```python
from build123d import *

# Parameters (mm, degrees)
SKETCH3_W           = 22
SKETCH3_H           = 5.7785
BOSS_EXTRUDE2_DEPTH = 101
CUT_EXTRUDE1_DEPTH  = 104.529662717
FILLET1_R           = 1.2637
SKETCH10_W          = 101
SKETCH10_H          = 62
BOSS_EXTRUDE6_DEPTH = 8
SKETCH11_R          = 2.5
CUT_EXTRUDE2_DEPTH  = 110.676797911
SKETCH12_R          = 2.5
CUT_EXTRUDE3_DEPTH  = 110.676797911


with BuildPart() as part:
    # Sketch3 → Boss-Extrude2 (new body)
    with BuildSketch(Plane(origin=(0, 0, 0), x_dir=(0, 0, -1), z_dir=(1, 0, 0))):
        with Locations((11, 2.88925)):
            Rectangle(SKETCH3_W, SKETCH3_H)
    extrude(amount=-BOSS_EXTRUDE2_DEPTH)

    # Sketch5 → Cut-Extrude1 (cut, through all)
    with BuildSketch(Plane(origin=(0, 0, 0), x_dir=(-1, 0, 0), z_dir=(0, 0, -1))):
        with BuildLine():
            Line((1.674138493, 2.258445519), (0.421264214, 6.934235985))
            Line((0.421264214, 6.934235985), (6.147128546, 6.934235985))
            Line((6.147128546, 6.934235985), (4.894261507, 2.258445519))
            ThreePointArc((4.894261507, 2.258445519), (4.454663567, 1.600540709), (3.7054, 1.3462))
            Line((3.7054, 1.3462), (2.863, 1.3462))
            ThreePointArc((2.863, 1.3462), (2.113736433, 1.600540709), (1.674138493, 2.258445519))
        make_face()
        with BuildLine():
            Line((10.263138493, 2.258445519), (9.010264214, 6.934235985))
            Line((9.010264214, 6.934235985), (14.736128546, 6.934235985))
            Line((14.736128546, 6.934235985), (13.483261507, 2.258445519))
            ThreePointArc((13.483261507, 2.258445519), (13.043663567, 1.600540709), (12.2944, 1.3462))
            Line((12.2944, 1.3462), (11.452, 1.3462))
            ThreePointArc((11.452, 1.3462), (10.702736433, 1.600540709), (10.263138493, 2.258445519))
        make_face()
        with BuildLine():
            Line((18.852138493, 2.258445519), (17.599264214, 6.934235985))
            Line((17.599264214, 6.934235985), (23.325128546, 6.934235985))
            Line((23.325128546, 6.934235985), (22.072261507, 2.258445519))
            ThreePointArc((22.072261507, 2.258445519), (21.632663567, 1.600540709), (20.8834, 1.3462))
            Line((20.8834, 1.3462), (20.041, 1.3462))
            ThreePointArc((20.041, 1.3462), (19.291736433, 1.600540709), (18.852138493, 2.258445519))
        make_face()
        with BuildLine():
            Line((27.441138493, 2.258445519), (26.188264214, 6.934235985))
            Line((26.188264214, 6.934235985), (31.914128546, 6.934235985))
            Line((31.914128546, 6.934235985), (30.661261507, 2.258445519))
            ThreePointArc((30.661261507, 2.258445519), (30.221663567, 1.600540709), (29.4724, 1.3462))
            Line((29.4724, 1.3462), (28.63, 1.3462))
            ThreePointArc((28.63, 1.3462), (27.880736433, 1.600540709), (27.441138493, 2.258445519))
        make_face()
        with BuildLine():
            Line((36.030138493, 2.258445519), (34.777264214, 6.934235985))
            Line((34.777264214, 6.934235985), (40.503128546, 6.934235985))
            Line((40.503128546, 6.934235985), (39.250261507, 2.258445519))
            ThreePointArc((39.250261507, 2.258445519), (38.810663567, 1.600540709), (38.0614, 1.3462))
            Line((38.0614, 1.3462), (37.219, 1.3462))
            ThreePointArc((37.219, 1.3462), (36.469736433, 1.600540709), (36.030138493, 2.258445519))
        make_face()
        with BuildLine():
            Line((44.619138493, 2.258445519), (43.366264214, 6.934235985))
            Line((43.366264214, 6.934235985), (49.092128546, 6.934235985))
            Line((49.092128546, 6.934235985), (47.839261507, 2.258445519))
            ThreePointArc((47.839261507, 2.258445519), (47.399663567, 1.600540709), (46.6504, 1.3462))
            Line((46.6504, 1.3462), (45.808, 1.3462))
            ThreePointArc((45.808, 1.3462), (45.058736433, 1.600540709), (44.619138493, 2.258445519))
        make_face()
        with BuildLine():
            Line((53.208138493, 2.258445519), (51.955264214, 6.934235985))
            Line((51.955264214, 6.934235985), (57.681128546, 6.934235985))
            Line((57.681128546, 6.934235985), (56.428261507, 2.258445519))
            ThreePointArc((56.428261507, 2.258445519), (55.988663567, 1.600540709), (55.2394, 1.3462))
            Line((55.2394, 1.3462), (54.397, 1.3462))
            ThreePointArc((54.397, 1.3462), (53.647736433, 1.600540709), (53.208138493, 2.258445519))
        make_face()
        with BuildLine():
            Line((61.797138493, 2.258445519), (60.544264214, 6.934235985))
            Line((60.544264214, 6.934235985), (66.270128546, 6.934235985))
            Line((66.270128546, 6.934235985), (65.017261507, 2.258445519))
            ThreePointArc((65.017261507, 2.258445519), (64.577663567, 1.600540709), (63.8284, 1.3462))
            Line((63.8284, 1.3462), (62.986, 1.3462))
            ThreePointArc((62.986, 1.3462), (62.236736433, 1.600540709), (61.797138493, 2.258445519))
        make_face()
        with BuildLine():
            Line((70.386138493, 2.258445519), (69.133264214, 6.934235985))
            Line((69.133264214, 6.934235985), (74.859128546, 6.934235985))
            Line((74.859128546, 6.934235985), (73.606261507, 2.258445519))
            ThreePointArc((73.606261507, 2.258445519), (73.166663567, 1.600540709), (72.4174, 1.3462))
            Line((72.4174, 1.3462), (71.575, 1.3462))
            ThreePointArc((71.575, 1.3462), (70.825736433, 1.600540709), (70.386138493, 2.258445519))
        make_face()
        with BuildLine():
            Line((78.975138493, 2.258445519), (77.722264214, 6.934235985))
            Line((77.722264214, 6.934235985), (83.448128546, 6.934235985))
            Line((83.448128546, 6.934235985), (82.195261507, 2.258445519))
            ThreePointArc((82.195261507, 2.258445519), (81.755663567, 1.600540709), (81.0064, 1.3462))
            Line((81.0064, 1.3462), (80.164, 1.3462))
            ThreePointArc((80.164, 1.3462), (79.414736433, 1.600540709), (78.975138493, 2.258445519))
        make_face()
        with BuildLine():
            Line((87.564138493, 2.258445519), (86.311264214, 6.934235985))
            Line((86.311264214, 6.934235985), (92.037128546, 6.934235985))
            Line((92.037128546, 6.934235985), (90.784261507, 2.258445519))
            ThreePointArc((90.784261507, 2.258445519), (90.344663567, 1.600540709), (89.5954, 1.3462))
            Line((89.5954, 1.3462), (88.753, 1.3462))
            ThreePointArc((88.753, 1.3462), (88.003736433, 1.600540709), (87.564138493, 2.258445519))
        make_face()
        with BuildLine():
            Line((96.153138493, 2.258445519), (94.900264214, 6.934235985))
            Line((94.900264214, 6.934235985), (100.626128546, 6.934235985))
            Line((100.626128546, 6.934235985), (99.373261507, 2.258445519))
            ThreePointArc((99.373261507, 2.258445519), (98.933663567, 1.600540709), (98.1844, 1.3462))
            Line((98.1844, 1.3462), (97.342, 1.3462))
            ThreePointArc((97.342, 1.3462), (96.592736433, 1.600540709), (96.153138493, 2.258445519))
        make_face()
    extrude(amount=CUT_EXTRUDE1_DEPTH, mode=Mode.SUBTRACT)

    # Fillet1
    # the kernel refuses this fillet: 1.2637 mm, written as the material it takes off along each edge
    with BuildSketch(Plane(origin=(-14.426451812, 5.7785, -24.424181413), x_dir=(-1, 0, 0), z_dir=(0, 0, 1)), Plane(origin=(-23.015451812, 5.7785, -24.424181413), x_dir=(-1, 0, 0), z_dir=(0, 0, 1)), Plane(origin=(-31.604451812, 5.7785, -24.424181413), x_dir=(-1, 0, 0), z_dir=(0, 0, 1)), Plane(origin=(-40.193451812, 5.7785, -24.424181413), x_dir=(-1, 0, 0), z_dir=(0, 0, 1)), Plane(origin=(-48.782451812, 5.7785, -24.424181413), x_dir=(-1, 0, 0), z_dir=(0, 0, 1)), Plane(origin=(-57.371451812, 5.7785, -24.424181413), x_dir=(-1, 0, 0), z_dir=(0, 0, 1)), Plane(origin=(-65.960451812, 5.7785, -24.424181413), x_dir=(-1, 0, 0), z_dir=(0, 0, 1)), Plane(origin=(-74.549451812, 5.7785, -24.424181413), x_dir=(-1, 0, 0), z_dir=(0, 0, 1)), Plane(origin=(-83.138451812, 5.7785, -24.424181413), x_dir=(-1, 0, 0), z_dir=(0, 0, 1)), Plane(origin=(-91.727451812, 5.7785, -24.424181413), x_dir=(-1, 0, 0), z_dir=(0, 0, 1)), Plane(origin=(-5.837451812, 5.7785, -24.424181413), x_dir=(-1, 0, 0), z_dir=(0, 0, 1))) as fillet1_piece_1:
        with BuildLine():
            CenterArc((FILLET1_R * 0.767328135667, FILLET1_R), FILLET1_R, 194.999917223, 75.000082777)
            Line((-FILLET1_R * 0.198598064545, FILLET1_R * 0.7411823504), (-FILLET1_R * 0.217916588549, FILLET1_R * 0.736005997408))
            Line((-FILLET1_R * 0.217916588549, FILLET1_R * 0.736005997408), (-FILLET1_R * 0.0153465627133, -FILLET1_R * 0.02))
            Line((-FILLET1_R * 0.0153465627133, -FILLET1_R * 0.02), (FILLET1_R * 0.767328135667, -FILLET1_R * 0.02))
            Line((FILLET1_R * 0.767328135667, -FILLET1_R * 0.02), (FILLET1_R * 0.767328135667, 0))
        make_face()
    extrude(amount=26.848362825, mode=Mode.SUBTRACT)
    with BuildSketch(Plane(origin=(-9.319942738, 5.7785, 2.424177787), x_dir=(-0.25881904510252474, -0.9659258262890672, 0), z_dir=(0, 0, -1)), Plane(origin=(-17.908942738, 5.7785, 2.424177787), x_dir=(-0.25881904510252474, -0.9659258262890672, 0), z_dir=(0, 0, -1)), Plane(origin=(-26.497942738, 5.7785, 2.424177787), x_dir=(-0.25881904510252496, -0.9659258262890672, 0), z_dir=(0, 0, -1)), Plane(origin=(-35.086942738, 5.7785, 2.424177787), x_dir=(-0.2588190451025256, -0.965925826289067, 0), z_dir=(0, 0, -1)), Plane(origin=(-43.675942738, 5.7785, 2.424177787), x_dir=(-0.2588190451025256, -0.965925826289067, 0), z_dir=(0, 0, -1)), Plane(origin=(-52.264942738, 5.7785, 2.424177787), x_dir=(-0.25881904510252424, -0.9659258262890673, 0), z_dir=(0, 0, -1)), Plane(origin=(-60.853942738, 5.7785, 2.424177787), x_dir=(-0.25881904510252424, -0.9659258262890673, 0), z_dir=(0, 0, -1)), Plane(origin=(-69.442942738, 5.7785, 2.424177787), x_dir=(-0.25881904510252607, -0.9659258262890669, 0), z_dir=(0, 0, -1)), Plane(origin=(-78.031942738, 5.7785, 2.424177787), x_dir=(-0.25881904510252607, -0.9659258262890669, 0), z_dir=(0, 0, -1)), Plane(origin=(-86.620942738, 5.7785, 2.424177787), x_dir=(-0.2588190451025252, -0.9659258262890671, 0), z_dir=(0, 0, -1)), Plane(origin=(-95.209942738, 5.7785, 2.424177787), x_dir=(-0.2588190451025268, -0.9659258262890666, 0), z_dir=(0, 0, -1))) as fillet1_piece_2:
        with BuildLine():
            CenterArc((FILLET1_R * 0.767326987979, -FILLET1_R), FILLET1_R, 90, 75)
            Line((-FILLET1_R * 0.19859883831, -FILLET1_R * 0.741180954897), (-FILLET1_R * 0.217917354836, -FILLET1_R * 0.736004573995))
            Line((-FILLET1_R * 0.217917354836, -FILLET1_R * 0.736004573995), (-FILLET1_R * 0.0153465397596, FILLET1_R * 0.02))
            Line((-FILLET1_R * 0.0153465397596, FILLET1_R * 0.02), (FILLET1_R * 0.767326987979, FILLET1_R * 0.02))
            Line((FILLET1_R * 0.767326987979, FILLET1_R * 0.02), (FILLET1_R * 0.767326987979, 0))
        make_face()
    extrude(amount=26.848355574, mode=Mode.SUBTRACT)
    with BuildSketch(Plane(origin=(-100.316451812, 5.7785, -24.33349599), x_dir=(-1, 0, 0), z_dir=(0, 0, 1))) as fillet1_piece_3:
        with BuildLine():
            CenterArc((0.97906096, 1.22866183), FILLET1_R, 194.999917223, 61.476400821)
            Line((-0.241579979, 0.901593966), (-0.265992798, 0.895052609))
            Line((-0.265992798, 0.895052609), (-0.024412819, -0.006541357))
            Line((-0.024412819, -0.006541357), (0, -0.025274))
            ThreePointArc((0, -0.025274), (0.341774094, -0.025274), (0.677637933, -0.024573237))
            Line((0.677637933, -0.024573237), (0.683548188, 0))
        make_face()
    extrude(amount=26.666991979, mode=Mode.SUBTRACT)
    with BuildSketch(Plane(origin=(-0.730942738, 5.7785, 2.362037613), x_dir=(-0.2588190451025249, -0.9659258262890672, 0), z_dir=(0, 0, -1))) as fillet1_piece_4:
        with BuildLine():
            CenterArc((0.944815045, -1.2637), FILLET1_R, 90, 63.813512011)
            Line((-0.189181901, -0.706036468), (-0.21186184, -0.694883197))
            ThreePointArc((-0.21186184, -0.694883197), (-0.11900376, -0.346476841), (-0.024412809, 0.006541393))
            Line((-0.024412809, 0.006541393), (0, 0.025274))
            Line((0, 0.025274), (0.944815045, 0.025274))
            Line((0.944815045, 0.025274), (0.944815045, 0))
        make_face()
    extrude(amount=26.724075226, mode=Mode.SUBTRACT)

    # Sketch10 → Boss-Extrude6 (add)
    with BuildSketch(Plane(origin=(0, 0, 0), x_dir=(1, 0, 0), z_dir=(0, 1, 0))):
        with Locations((-50.5, 11)):
            Rectangle(SKETCH10_W, SKETCH10_H)
    extrude(amount=-BOSS_EXTRUDE6_DEPTH)

    # Sketch11 → Cut-Extrude2 (cut, through all)
    with BuildSketch(Plane(origin=(0, 0, 0), x_dir=(1, 0, 0), z_dir=(0, 1, 0))):
        with Locations(Location((-8.5, -10, 0), (0, 0, 270))):
            Circle(SKETCH11_R)
        with Locations(Location((-92.5, -10, 0), (0, 0, 270))):
            Circle(SKETCH11_R)
    extrude(amount=-CUT_EXTRUDE2_DEPTH, mode=Mode.SUBTRACT)

    # Sketch12 → Cut-Extrude3 (cut, through all)
    with BuildSketch(Plane(origin=(0, 0, 0), x_dir=(1, 0, 0), z_dir=(0, 1, 0))):
        with Locations(Location((-8.5, 32, 0), (0, 0, 270))):
            Circle(SKETCH12_R)
        with Locations(Location((-92.5, 32, 0), (0, 0, 270))):
            Circle(SKETCH12_R)
    extrude(amount=-CUT_EXTRUDE3_DEPTH, mode=Mode.SUBTRACT)


solid = part.part
```
The listing builds one solid part. Answer for the finished solid, in the listing's coordinates (mm). A direction names the side the tool comes from. Coordinates: 2 decimals unless noted, no trailing zeros. Loops run counter-clockwise (first coordinate to the right, second up) from the corner with the lowest first, then second, coordinate; pieces in that order, holes last. Notation, with made-up numbers: (-27, 71) - (-7, 71) arc R11 cw to (-7, 81) - close; hole circle Ø10 at (42.25, -23.75). An arc over 180 degrees is marked (long way). Use a Markdown table: item, result. Add a question column.
1) The part is cut by section B-B, the plane z = 14.5. Give the vertices of the cut face in (x, y).
2) Given pin 1 (0.9 mm diameter, centred on x = -3.5, z = -8, fed in from +Y); pin 2 (4.5 mm diameter, centred on x = -8.5, z = 10, fed in from +Y); pin 3 (22 mm diameter, centred on x = -54, z = 14.5, fed in from +Y); pin 4 (4.5 mm diameter, centred on x = -37.5, y = 1.5, fed in from +Z), each flat-ended and moving along its own axis, determine where each tip first touches the part or whether it passes through.
3) The mould has two halves that part along X. Classify faces 1 (the flat face through (-73.957, 3.568, -10.846)), 2 (the flat face through (-101, -3, -11)), 3 (the cylindrical face through (-10.94, -3.94, 9.46)), 4 (the flat face through (-51, 0, 10)): released by +X, released by -X, zero draft, split by the parting line, or undercut.
4) For faces 5 (the flat face through (-51, -8, -11)), 6 (the flat face through (-51, 0, -32)), 7 (the flat face through (-31.012, 3.568, -10.846)), determine the directions among +Z, -Z, +X, -X, +Y, -Y from which every point of the face is accessible in a straight line to the end or side of a thin tool.
5) Find the intervals of material crossed by line 1 (X direction, y = -4, z = -32); line 2 (X direction, y = -6.25, z = 10.5); line 3 (Y direction, x = -49.5, z = 4), in increasing order.
6) The part is cut by section A-A, the plane z = -32. Give the vertices of the cut face in (x, y).
Here are the results:
| question | item | result |
|---|---|---|
| 1 | outline | (-101, -8) - (0, -8) - (0, 0) - (-101, 0) - close |
| 2 | pin 1 | stops at y = 1.37 |
| 2 | pin 2 | passes through |
| 2 | pin 3 | stops at y = 0 |
| 2 | pin 4 | stops at z = 20 |
| 3 | face 1 | undercut |
| 3 | face 2 | released by -X |
| 3 | face 3 | undercut |
| 3 | face 4 | zero draft |
| 4 | face 5 | +Z, -Z, +X, -X, -Y |
| 4 | face 6 | -Z, +X, -X, +Y |
| 4 | face 7 | +Z, -Z, +Y |
| 5 | line 1 | x = -101 to -95, -90 to -11, -6 to 0 |
| 5 | line 2 | x = -101 to -94.95, -90.05 to -10.95, -6.05 to 0 |
| 5 | line 3 | y = -8 to 0 |
| 6 | outline | (-101, -8) - (-95, -8) - (-95, 0) - (-101, 0) - close; (-90, -8) - (-11, -8) - (-11, 0) - (-90, 0) - close; (-6, -8) - (0, -8) - (0, 0) - (-6, 0) - close |
